Geometry check sheet. Reference: drawing and pictorial views, mm from the part's lowest x, y, z. A direction names the side the tool comes from. Round coordinates to 2 decimals unless told otherwise and drop trailing zeros. Order: outer loops, then holes, each group sorted by start corner. A loop starts at its lowest first (then second) coordinate and runs counter-clockwise, first axis right, second up.
Q1. Cross-section at A-A on z = 7.5. Record the cut outline in (x, y).
Q2. Scan lines: probe 1 along Z at (x, y) = (5.85, 6.5); probe 2 along Y at (x, z) = (0.5, 8); probe 3 along Y at (x, z) = (6.2, 7.5). Record each from-to range of solid material in increasing order.
Q3. Set-up check for the marked faces 5, 6 and 7: record each of +Z, -Z, +X, -X, +Y, -Y from which the full face is reachable in a straight line by a thin tool's end or side.
Q4. Cross-section at C-C on x = 2.5. Record the cut outline in (y, z) (1 decimal).
Q5. Depth check by flat-ended pin: P1, Ø2, axis at y = 7.5, z = 4.5, coming from the +X side. Enter the tip coordinate at first touch or a pass-through.
Q6. Cross-section at D-D on x = 6.25. Record the cut outline in (y, z).
Q7. Mould release check, pull along Z, two halves, no side actions. Record for the marked faces 1, 2, 3 and 4: +Z half, -Z half, draft (parallel to the pull), parting line (faces both ways), or undercut.
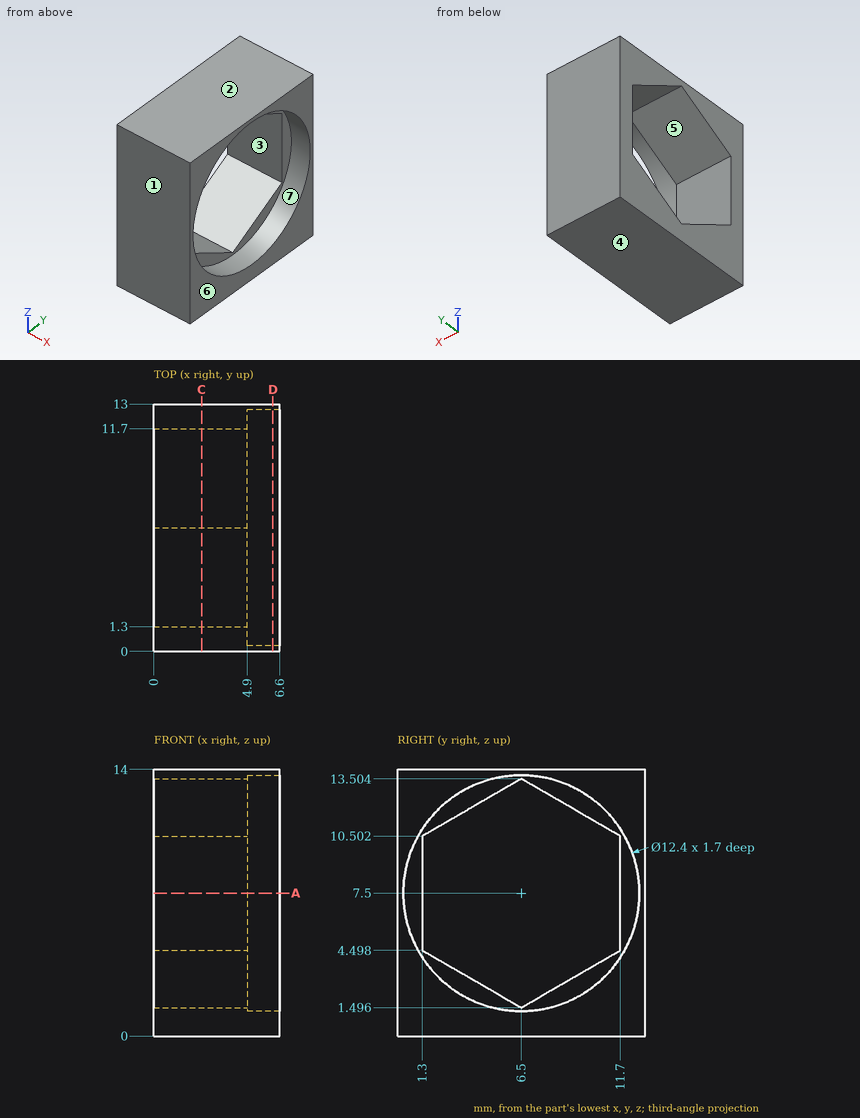
Results found:
1. outline: (0, 0) - (6.6, 0) - (6.6, 0.3) - (4.9, 0.3) - (4.9, 1.3) - (0, 1.3) - close; (0, 11.7) - (4.9, 11.7) - (4.9, 12.7) - (6.6, 12.7) - (6.6, 13) - (0, 13) - close
2. probe 1: z = 0 to 1.3, 13.7 to 14
2. probe 2: y = 0 to 1.3, 11.7 to 13
2. probe 3: y = 0 to 0.3, 12.7 to 13
3. face 5: +X, -X
3. face 6: +Z, -Z, +X, +Y, -Y
3. face 7: +X
4. outline: (0, 0) - (13, 0) - (13, 14) - (0, 14) - close; hole (1.3, 4.5) - (6.5, 1.5) - (11.7, 4.5) - (11.7, 10.5) - (6.5, 13.5) - (1.3, 10.5) - close
5. P1: passes through
6. outline: (0, 0) - (13, 0) - (13, 14) - (0, 14) - close; hole circle Ø12.4 at (6.5, 7.5)
7. face 1: draft
7. face 2: +Z half
7. face 3: undercut
7. face 4: -Z half
